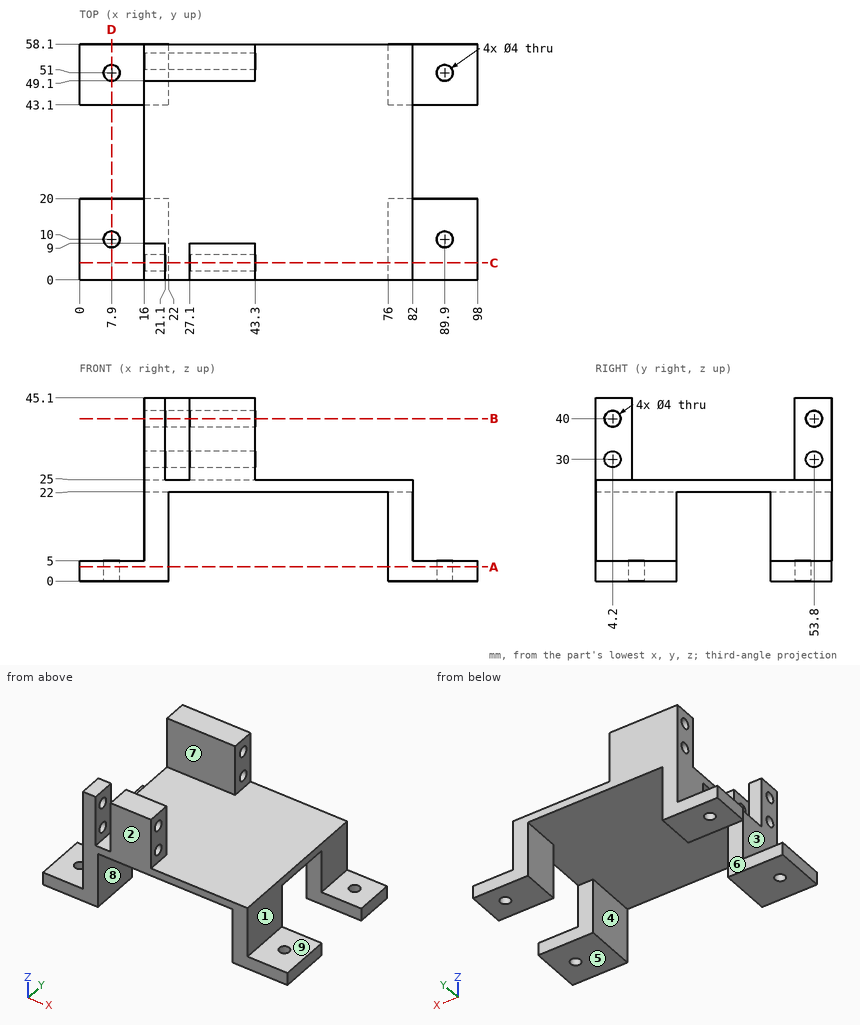
Geometry: see drawing. Coordinates: mm, zero at the bounding-box minimum. A direction names the side the tool comes from. Round coordinates to 2 decimals unless told otherwise and drop trailing zeros. Write each loop counter-clockwise with the first axis right and the second up, starting at its lowest first coordinate (ties: lowest second). Pieces come first, ordered by that corner, then holes. Notation, with made-up numbers: M -16,-24.5 L 15,-24.5 A21 cw 15,3.5 Z; hole C 19,51.5 d5. An arc over 180 degrees is marked long. Answer as a JSON object with one key per item and string values. Group by question number.
(1) Section query D-D on x = 7.9. Output: boundary loops of the cut face in (y, z), then the cut area to 3 significant figures.
(2) Mould query, pull axis X, two halves, no side actions, for the marked faces 1, 2, 3 and 4. Classes: +X half, -X half, draft (parallel to the pull), parting line (faces both ways), or undercut.
(3) Reachability of the marked faces 5, 6, 7, 8 and 9 from +Z, -Z, +X, -X, +Y, -Y: full face, straight path, thin tool, end or side. Return the list, or none.
(4) Section query B-B on z = 40. Output: boundary loops of the cut face in (x, y).
(5) Section query C-C on y = 4.2. State how many separate pieces and enclosed holes the cut face has, then the cut area to 3 significant figures.
(6) Section query A-A on z = 3.5. Output: boundary loops of the cut face in (x, y), then the cut area to 3 significant figures.
(7) First-contact query: pin 1 (5 mm diameter, centred on y = 53.8, z = 40, fed in from +X); pin 2 (8 mm diameter, centred on x = 5, y = 7, fed in from +Z); pin 3 (2.5 mm diameter, centred on y = 2.5, z = 39.5, fed in from -X); pin 4 (22 mm diameter, centred on y = 9, z = 15.5, fed in from +X). Flat tips, straight axial feed; report the tip coordinate or a pass-through.
(8) Ray query, line 1 (X direction, y = 10, z = 3.6); line 2 (Y direction, x = 18.35, z = 40); line 3 (Y direction, x = 89.9, z = 3.9). Return the intervals inside material, ascending. Write a range as [from, to].
Computed values:
{
 "1": {"outline": "M 0,0 L 8,0 L 8,5 L 0,5 Z; M 12,0 L 20,0 L 20,5 L 12,5 Z; M 43.1,0 L 49,0 L 49,5 L 43.1,5 Z; M 53,0 L 58.1,0 L 58.1,5 L 53,5 Z", "area": "135 mm^2"},
 "2": {"face 1": "+X half", "face 2": "draft", "face 3": "-X half", "face 4": "undercut"},
 "3": {"face 5": "-Z, +X, -X, +Y, -Y", "face 6": "-Z, +X, -X", "face 7": "+Z, +X, -X", "face 8": "-Z, +Y, -Y", "face 9": "+Z, +X, +Y, -Y"},
 "4": {"outline": "M 16,0 L 21.1,0 L 21.1,2.2 L 16,2.2 Z; M 16,6.2 L 21.1,6.2 L 21.1,9 L 16,9 Z; M 16,49.1 L 43.3,49.1 L 43.3,51.8 L 16,51.8 Z; M 16,55.8 L 43.3,55.8 L 43.3,58.1 L 16,58.1 Z; M 27.1,0 L 43.3,0 L 43.3,2.2 L 27.1,2.2 Z; M 27.1,6.2 L 43.3,6.2 L 43.3,9 L 27.1,9 Z"},
 "5": {"separate pieces": "5", "enclosed holes": "0", "area": "880 mm^2"},
 "6": {"outline": "M 0,0 L 22,0 L 22,20 L 0,20 Z; M 0,43.1 L 22,43.1 L 22,58.1 L 0,58.1 Z; M 76,0 L 98,0 L 98,20 L 76,20 Z; M 76,43.1 L 98,43.1 L 98,58.1 L 76,58.1 Z; hole C 7.9,10 d4; hole C 7.9,51 d4; hole C 89.9,10 d4; hole C 89.9,51 d4", "area": "1,490 mm^2"},
 "7": {"pin 1": "x = 43.3", "pin 2": "z = 5", "pin 3": "x = 16", "pin 4": "x = 98"},
 "8": {"line 1": "[0, 5.9], [9.9, 22], [76, 87.9], [91.9, 98]", "line 2": "[0, 2.2], [6.2, 9], [49.1, 51.8], [55.8, 58.1]", "line 3": "[0, 8], [12, 20], [43.1, 49], [53, 58.1]"}
}
